Part model, mm, in its own coordinate system. A direction names the side the tool comes from. Round coordinates to 2 decimals unless told otherwise and drop trailing zeros. Loops run counter-clockwise (first coordinate to the right, second up) from the corner with the lowest first, then second, coordinate; pieces in that order, holes last. Notation, with made-up numbers: (27, 26.25) -> (55, 26.25) arc R16 cw to (55, 43.25) -> close; hole circle Ø1 at (-28, -23.5). An arc over 180 degrees is marked (long way). Answer as CSV lines item,"result".
from build123d import *

# Parameters (mm, degrees)
BOSS_EXTRUDE1_DEPTH       = 8
CUT_EXTRUDE2_DEPTH        = 20.5
SKETCH6_W                 = 35.270415117
SKETCH6_H                 = 22.226622545
CUT_EXTRUDE3_DEPTH        = 8
BOSS_EXTRUDE2_DEPTH       = 3
BOSS_EXTRUDE7_DEPTH       = 5
SKETCH7_R                 = 1.6
CUT_EXTRUDE6_DEPTH        = 40.255572853
F_3_0MM_DOWEL_HOLE1_D     = 3
F_3_0MM_DOWEL_HOLE1_DEPTH = 5
F_3_0MM_DOWEL_HOLE1_TIP   = 0.901290929


with BuildPart() as part:
    # Sketch1 → Boss-Extrude1 (new body)
    with BuildSketch(Plane(origin=(0, 0, 0), x_dir=(0, 0, -1), z_dir=(1, 0, 0))):
        Polygon((0, 0), (0, 16), (-3.5, 16), (-3.5, 4), (-24, 4), (-24, 18), (-31, 18), (-31, 0), align=None)
    boss_extrude1 = extrude(amount=-BOSS_EXTRUDE1_DEPTH)

    # Sketch5 → Cut-Extrude2 (cut)
    with BuildSketch(Plane.XY.offset(3.5)):
        Polygon((-8, 0), (-3, 0), (-5, 4), (-8, 4), align=None)
    cut_extrude2 = extrude(amount=CUT_EXTRUDE2_DEPTH, mode=Mode.SUBTRACT)

    # Mirror1: Boss-Extrude1, Cut-Extrude2 across plane
    add(boss_extrude1.mirror(Plane(origin=(-8, 0, 0), x_dir=(0, 0, 1), z_dir=(1, 0, 0))))
    add(cut_extrude2.mirror(Plane(origin=(-8, 0, 0), x_dir=(0, 0, 1), z_dir=(1, 0, 0))), mode=Mode.SUBTRACT)

    # Sketch6 → Cut-Extrude3 (cut)
    with BuildSketch(Plane(origin=(0, 0, 0), x_dir=(0, 0, -1), z_dir=(1, 0, 0))):
        with Locations((-16.260875851, 8.713036563)):
            Rectangle(SKETCH6_W, SKETCH6_H)
    extrude(amount=-CUT_EXTRUDE3_DEPTH, mode=Mode.SUBTRACT)

    # Sketch9 → Boss-Extrude2 (add)
    with BuildSketch(Plane.XY.offset(3.5)):
        Polygon((-11, 4), (-13, 0), (-8, 0), (-8, 4), align=None)
    extrude(amount=BOSS_EXTRUDE2_DEPTH)

    # Sketch13 → Boss-Extrude7 (add)
    with BuildSketch(Plane.XZ):
        with BuildLine():
            Line((-14, 33), (-6, 33))
            Line((-6, 33), (-6, 26))
            ThreePointArc((-6, 26), (-6.585786438, 24.585786438), (-8, 24))
            Line((-8, 24), (-8, 31))
            Line((-8, 31), (-16, 31))
            ThreePointArc((-16, 31), (-15.414213562, 32.414213562), (-14, 33))
        make_face()
    extrude(amount=-BOSS_EXTRUDE7_DEPTH)

    # Sketch7 → Cut-Extrude6 (cut, through all)
    with BuildSketch(Plane.XY.offset(31)):
        with Locations((-12, 12)):
            Circle(SKETCH7_R)
    extrude(amount=-CUT_EXTRUDE6_DEPTH, mode=Mode.SUBTRACT)

    # Ø3.0mm Dowel Hole1
    with Locations(Plane(origin=(0, 0, 0), x_dir=(-1, 0, 0), z_dir=(0, -1, 0))):
        with Locations((10.285, -29)):
            Hole(F_3_0MM_DOWEL_HOLE1_D / 2, depth=F_3_0MM_DOWEL_HOLE1_DEPTH)
            with Locations((0, 0, -(F_3_0MM_DOWEL_HOLE1_DEPTH + F_3_0MM_DOWEL_HOLE1_TIP / 2))):  # 118° drill point
                Cone(0, F_3_0MM_DOWEL_HOLE1_D / 2, F_3_0MM_DOWEL_HOLE1_TIP, mode=Mode.SUBTRACT)


solid = part.part
Q1. Two-plate mould, pull along Z, no slides. Class faces 4 (the face through (-12, 9, 24)), 5 (the face through (-6, 2, 30)), 6 (the face through (-12, 10, 31)): pulls with the +Z half, pulls with the -Z half, needs draft (parallel to the pull), parting line crosses it, or undercut.
Geometry results:
face 4,"undercut"
face 5,"needs draft"
face 6,"pulls with the +Z half"
Q2. Saw through at B-B, the plane z = 2. Write the cut outline in (x, y), then the cut area to 3 significant figures.
Geometry results:
outline,"(-16, 0) -> (-8, 0) -> (-8, 16) -> (-16, 16) -> close; hole circle Ø3.2 at (-12, 12)"
area,"120 mm2"
Q3. Saw through at D-D, the plane y = 2.5. Write the cut outline in (x, z) (3 decimals), then the cut area to 3 significant figures.
Geometry results:
outline,"(-16, 0) -> (-8, 0) -> (-8, 6.5) -> (-11.75, 6.5) -> (-11.75, 24) -> (-8, 24) arc R2 ccw to (-6, 26) -> (-6, 33) -> (-14, 33) arc R2 ccw to (-16, 31) -> close; hole circle Ø3 at (-10.285, 29)"
area,"208 mm2"
Q4. Saw through at A-A, the plane y = 12. Write the cut outline in (x, z), then the cut area to 3 significant figures.
Geometry results:
outline,"(-16, 0) -> (-13.6, 0) -> (-13.6, 3.5) -> (-16, 3.5) -> close; (-16, 24) -> (-13.6, 24) -> (-13.6, 31) -> (-16, 31) -> close; (-10.4, 0) -> (-8, 0) -> (-8, 3.5) -> (-10.4, 3.5) -> close; (-10.4, 24) -> (-8, 24) -> (-8, 31) -> (-10.4, 31) -> close"
area,"50.4 mm2"
Q5. Drill centre lines: line 1 along Y through (x, z) = (-12, 28); line 2 along Z through (x, y) = (-12, 14.75); line 3 along Z through (x, y) = (-12.75, 17). Where is each one in solid material? Low to high.
Geometry results:
line 1,"0 to 10.4, 13.6 to 18"
line 2,"0 to 3.5, 24 to 31"
line 3,"24 to 31"
Q6. Saw through at C-C, the plane y = 14. Write the cut outline in (x, z).
Geometry results:
outline,"(-16, 0) -> (-8, 0) -> (-8, 3.5) -> (-16, 3.5) -> close; (-16, 24) -> (-8, 24) -> (-8, 31) -> (-16, 31) -> close"
Q7. Drop flat-ended pins along their axis: P1, Ø3, axis at x = -12, y = 12, coming from the +Z side; P2, Ø5, axis at y = 5.5, z = 4, coming from the +X side; P3, Ø1, axis at x = -10.5, z = 1.5, coming from the +Y side; P4, Ø2.5, axis at x = -12.5, y = 7, coming from the +Z side. Give the stop position or say it passes through.
Geometry results:
P1,"through"
P2,"x = -8"
P3,"y = 16"
P4,"z = 31"
Q8. Which spindle directions (+Z, -Z, +X, -X, +Y, -Y) get a long thin tool onto all of the face, cutting with end or side? Do faces 1 (the face through (-8, 12, 28)), 2 (the face through (-8, 6, 2)), 3 (the face through (-13, 4, 14)). Say none if no direction does.
Geometry results:
face 1,"+Z, -Z, +X, +Y"
face 2,"-Z, +X, +Y, -Y"
face 3,"+X, -X, +Y"
